Could you check a few things on this drawing? It's one solid part, dimensions in mm from its lowest x, y, z. Coordinates: 2 decimals unless noted, no trailing zeros. Write each loop counter-clockwise with the first axis right and the second up, starting at its lowest first coordinate (ties: lowest second). Pieces come first, ordered by that corner, then holes.
Item 1: I want a section at D-D (z = 87). Please give me the cut outline in (x, y).
Item 2: If we mould it in two halves opening along Z, with no side actions, what happens to the marked faces 1, 2 and 3? For each: pulls with the +Z half, pulls with the -Z half, needs draft (parallel to the pull), parting line crosses it, or undercut.
Item 3: I'm going to push flat-ended pins straight in: P1, Ø1.5, axis at y = 9, z = 14.5, coming from the +X side; P2, Ø10, axis at x = 49.5, y = 25, coming from the -Z side; P3, Ø3, axis at y = 11.5, z = 55.5, coming from the -X side; P4, Ø1, axis at x = 12.5, z = 86.5, coming from the +Y side. Where does each tip first touch, or does it pass through?
Item 4: Please list where these lines run through material, in increasing order: line 1 (X direction, y = 19, z = 56.5); line 2 (Y direction, x = 18, z = 31.5); line 3 (X direction, y = 13.5, z = 66).
Item 5: I want a section at B-B (y = 24.75). Please give me the cut outline in (x, z), and give its area (3 significant figures).
Item 6: I want a section at C-C (x = 83). Please give me the cut outline in (y, z).
Item 7: I want a section at A-A (z = 50.5). Please give me the cut outline in (x, y), and give its area (3 significant figures).
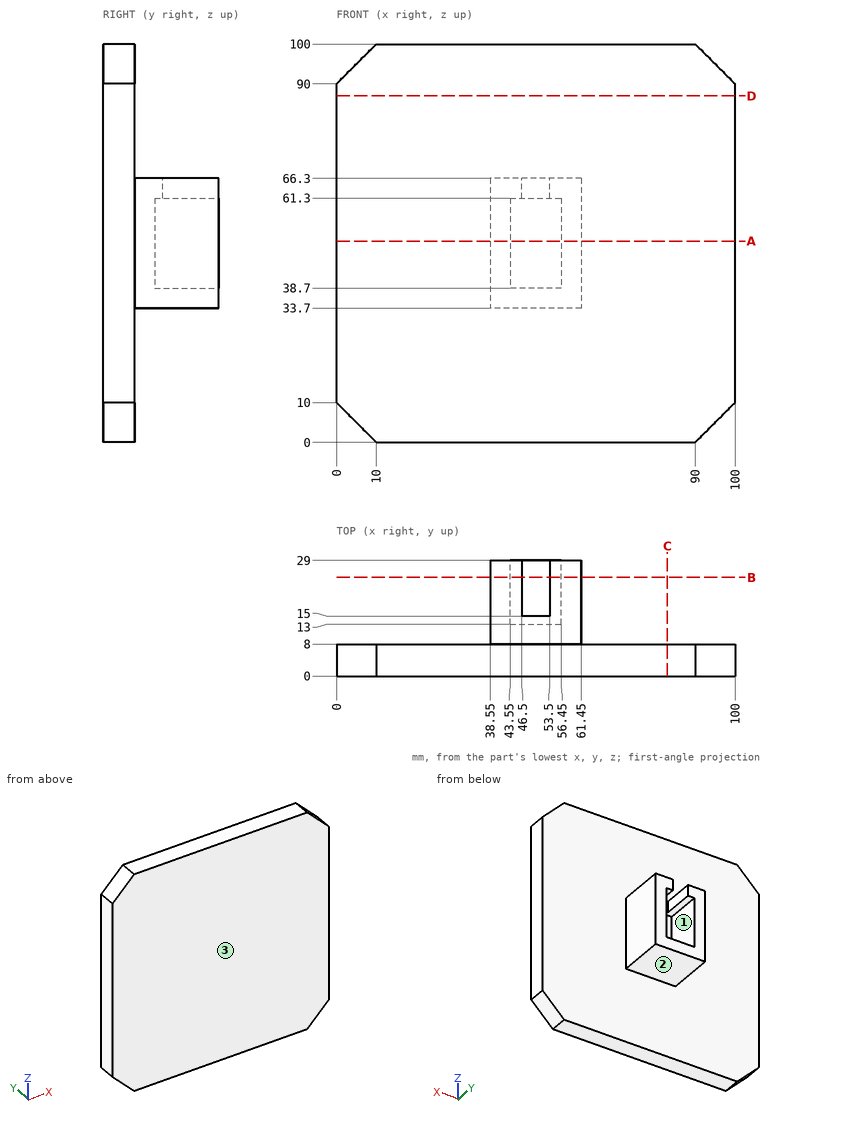
Answer:
1. outline: (0, 0) - (100, 0) - (100, 8) - (0, 8) - close
2. face 1: undercut
2. face 2: pulls with the -Z half
2. face 3: needs draft
3. P1: passes through
3. P2: stops at z = 33.7
3. P3: stops at x = 38.55
3. P4: stops at y = 8
4. line 1: x = 38.55 to 43.55, 56.45 to 61.45
4. line 2: y = 0 to 8
4. line 3: x = 38.55 to 61.45
5. outline: (38.55, 33.7) - (61.45, 33.7) - (61.45, 66.3) - (53.5, 66.3) - (53.5, 61.3) - (56.45, 61.3) - (56.45, 38.7) - (43.55, 38.7) - (43.55, 61.3) - (46.5, 61.3) - (46.5, 66.3) - (38.55, 66.3) - close
5. area: 420 mm2
6. outline: (0, 0) - (8, 0) - (8, 100) - (0, 100) - close
7. outline: (0, 0) - (100, 0) - (100, 8) - (61.45, 8) - (61.45, 29) - (56.45, 29) - (56.45, 13) - (43.55, 13) - (43.55, 29) - (38.55, 29) - (38.55, 8) - (0, 8) - close
7. area: 1,070 mm2
